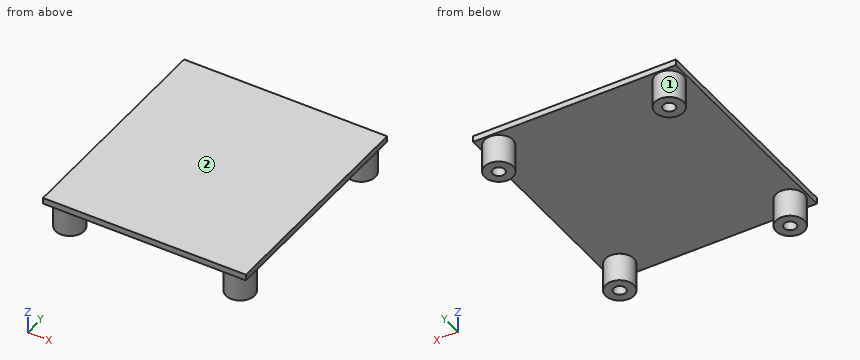
from build123d import *

# Parameters (mm, degrees)
SKETCH_1_W      = 50
SKETCH_1_H      = 56
EXTRUDE_1_DEPTH = 1.5
SKETCH_2_R      = 3.5
SKETCH_2_R_2    = 1.5
EXTRUDE_2_DEPTH = 7


with BuildPart() as part:
    # Эскиз1 → Бобышка-Вытянуть1 (new body)
    with BuildSketch(Plane.XY):
        with Locations((25, 28)):
            Rectangle(SKETCH_1_W, SKETCH_1_H)
    extrude(amount=EXTRUDE_1_DEPTH)

    # Эскиз2 → Бобышка-Вытянуть2 (add)
    # profile 1 of 4: a face of its own
    with BuildSketch(Plane(origin=(0, 0, 0), x_dir=(-1, 0, 0), z_dir=(0, 0, -1))):
        with Locations((-46, 52.2)):
            Circle(SKETCH_2_R)
        with Locations((-46, 52.2)):
            Circle(SKETCH_2_R_2, mode=Mode.SUBTRACT)
    # profile 2 of 4: a face of its own
    with BuildSketch(Plane(origin=(0, 0, 0), x_dir=(-1, 0, 0), z_dir=(0, 0, -1))):
        with Locations((-4, 52.2)):
            Circle(SKETCH_2_R)
        with Locations((-4, 52.2)):
            Circle(SKETCH_2_R_2, mode=Mode.SUBTRACT)
    # profile 3 of 4: a face of its own
    with BuildSketch(Plane(origin=(0, 0, 0), x_dir=(-1, 0, 0), z_dir=(0, 0, -1))):
        with Locations((-46, 4.2)):
            Circle(SKETCH_2_R)
        with Locations((-46, 4.2)):
            Circle(SKETCH_2_R_2, mode=Mode.SUBTRACT)
    # profile 4 of 4: a face of its own
    with BuildSketch(Plane(origin=(0, 0, 0), x_dir=(-1, 0, 0), z_dir=(0, 0, -1))):
        with Locations((-4, 4.2)):
            Circle(SKETCH_2_R)
        with Locations((-4, 4.2)):
            Circle(SKETCH_2_R_2, mode=Mode.SUBTRACT)
    extrude(amount=EXTRUDE_2_DEPTH)


solid = part.part
Build history of the part. All positions in model axes, mm. Face numbers are marked on the shaded views. Give positions to 0.01 mm unless a question says otherwise; leave off trailing zeros. Order: outer loops, then holes, each group sorted by start corner. A loop starts at its lowest first (then second) coordinate and runs counter-clockwise, first axis right, second up. Notation, with made-up numbers: M 2.5,-18.5 L 16.5,-18.5 A24 cw 16.5,14.5 Z; hole C 22.25,-4 d8. An arc over 180 degrees is marked long. Use one line per item in the form item = value.
1) Saw through at A-A (z = -4.5). Give the cut face in (x, y).
Calculated:
outline = C 4,4.2 d7; C 4,52.2 d7; C 46,4.2 d7; C 46,52.2 d7; hole C 4,4.2 d3; hole C 4,52.2 d3; hole C 46,4.2 d3; hole C 46,52.2 d3
2) Saw through at C-C (y = 52.2). Give the cut face in (x, z), plus the area to 3 significant figures.
Calculated:
outline = M 0,0 L 0.5,0 L 0.5,-7 L 2.5,-7 L 2.5,0 L 5.5,0 L 5.5,-7 L 7.5,-7 L 7.5,0 L 42.5,0 L 42.5,-7 L 44.5,-7 L 44.5,0 L 47.5,0 L 47.5,-7 L 49.5,-7 L 49.5,0 L 50,0 L 50,1.5 L 0,1.5 Z
area = 131 mm2
3) Two-plate mould, pull along X, no slides. Class the marked faces 1 and 2: released by +X, released by -X, zero draft, split by the parting line, or undercut.
Calculated:
face_1 = undercut
face_2 = zero draft
4) Saw through at D-D (y = 37). Give the cut face in (x, z), plus the area to 3 significant figures.
Calculated:
outline = M 0,0 L 50,0 L 50,1.5 L 0,1.5 Z
area = 75.0 mm2
5) Drop flat-ended pins along their axis: pin 1 (5 mm diameter, centred on x = 4, y = 52.2, fed in from -Z); pin 2 (15 mm diameter, centred on x = 22.5, y = 14.5, fed in from -Z); pin 3 (4 mm diameter, centred on x = 7.5, z = -4, fed in from +Y); pin 4 (2 mm diameter, centred on y = 49, z = -2.5, fed in from +X). Give the stop position or say it passes through.
Calculated:
pin_1 = -7
pin_2 = 0
pin_3 = 55.36
pin_4 = 48.72
6) Probe probe 1 along Y at (x, z) = (4, -1.75); probe 2 along Y at (x, z) = (5, -3.25); probe 3 along Y at (x, z) = (44, -6). List the from-to ranges inside material, lowest first.
Calculated:
probe_1 = 0.7 to 2.7, 5.7 to 7.7, 48.7 to 50.7, 53.7 to 55.7
probe_2 = 0.85 to 3.08, 5.32 to 7.55, 48.85 to 51.08, 53.32 to 55.55
probe_3 = 1.33 to 7.07, 49.33 to 55.07
7) Saw through at B-B (x = 4). Give the cut face in (y, z).
Calculated:
outline = M 0,0 L 0.7,0 L 0.7,-7 L 2.7,-7 L 2.7,0 L 5.7,0 L 5.7,-7 L 7.7,-7 L 7.7,0 L 48.7,0 L 48.7,-7 L 50.7,-7 L 50.7,0 L 53.7,0 L 53.7,-7 L 55.7,-7 L 55.7,0 L 56,0 L 56,1.5 L 0,1.5 Z
